Input: part model. Units: mm. Frame: model coordinates. Round coordinates to 2 decimals unless told otherwise and drop trailing zeros. Loops run counter-clockwise (first coordinate to the right, second up) from the corner with the lowest first, then second, coordinate; pieces in that order, holes last.
(1) Cut plane A-A, the plane y = 25. Output: boundary loops of the cut face in (x, z).
(2) First-contact query: pin 1 Ø4 at (y, z) = (25, 0) entering from -X; pin 2 Ø5 at (y, z) = (5, 0) entering from +X. Flat tips, straight axial feed; report the tip coordinate or a pass-through.
(3) Line query: line 1 (Y direction, x = 0, z = 4.25); line 2 (Y direction, x = -4.5, z = 0); line 3 (Z direction, x = 2.25, y = 66.5). Output: solid intervals per line, ascending.
(4) Cut plane C-C, the plane x = 0. Output: boundary loops of the cut face in (y, z), and give its area (3 significant figures).
(5) Cut plane B-B, the plane z = 0. Output: boundary loops of the cut face in (x, y), and give its area (3 significant figures).
(6) Cut plane D-D, the plane y = 114. Output: boundary loops of the cut face in (x, z).
from build123d import *

# Parameters (mm, degrees)
SKETCH_1_W          = 10
SKETCH_1_H          = 10
SKETCH_1_W_2        = 7
SKETCH_1_H_2        = 7
EXTRUDE_1_DEPTH     = 220
SKETCH_2_R          = 2.15
CUT_EXTRUDE_1_DEPTH = 221.283907719
SKETCH_3_R          = 2.15
CUT_EXTRUDE_2_DEPTH = 221.283907719


with BuildPart() as part:
    # ｽｹｯﾁ1 → 押し出し-薄板1 (new body)
    with BuildSketch(Plane(origin=(0, 0, 0), x_dir=(1, 0, 0), z_dir=(0, 1, 0))):
        Rectangle(SKETCH_1_W, SKETCH_1_H)
        Rectangle(SKETCH_1_W_2, SKETCH_1_H_2, mode=Mode.SUBTRACT)
    extrude(amount=EXTRUDE_1_DEPTH)

    # ｽｹｯﾁ2 → ｶｯﾄ - 押し出し1 (cut, through all)
    with BuildSketch(Plane.XY.offset(5)):
        with Locations((0, 205)):
            Circle(SKETCH_2_R)
        with Locations((0, 215)):
            Circle(SKETCH_2_R)
    extrude(amount=-CUT_EXTRUDE_1_DEPTH, mode=Mode.SUBTRACT)

    # ｽｹｯﾁ3 → ｶｯﾄ - 押し出し2 (cut, through all)
    with BuildSketch(Plane(origin=(5, 0, 0), x_dir=(0, 0, -1), z_dir=(1, 0, 0))):
        with Locations((0, 5)):
            Circle(SKETCH_3_R)
        with Locations((0, 25)):
            Circle(SKETCH_3_R)
    extrude(amount=-CUT_EXTRUDE_2_DEPTH, mode=Mode.SUBTRACT)


solid = part.part
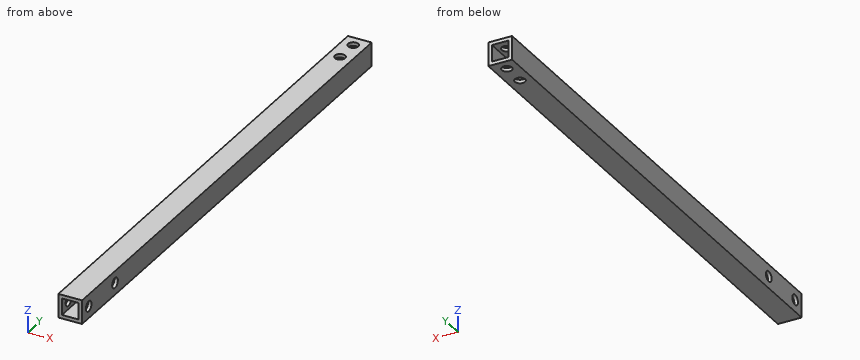
Reported:
1. outline: (-5, -5) - (5, -5) - (5, -2.15) - (3.5, -2.15) - (3.5, -3.5) - (-3.5, -3.5) - (-3.5, -2.15) - (-5, -2.15) - close; (-5, 2.15) - (-3.5, 2.15) - (-3.5, 3.5) - (3.5, 3.5) - (3.5, 2.15) - (5, 2.15) - (5, 5) - (-5, 5) - close
2. pin 1: passes through
2. pin 2: stops at x = 5
3. line 1: y = 0 to 202.85, 207.15 to 212.85, 217.15 to 220
3. line 2: y = 0 to 2.85, 7.15 to 22.85, 27.15 to 220
3. line 3: z = -5 to -3.5, 3.5 to 5
4. outline: (0, -5) - (202.85, -5) - (202.85, -3.5) - (0, -3.5) - close; (0, 3.5) - (202.85, 3.5) - (202.85, 5) - (0, 5) - close; (207.15, -5) - (212.85, -5) - (212.85, -3.5) - (207.15, -3.5) - close; (207.15, 3.5) - (212.85, 3.5) - (212.85, 5) - (207.15, 5) - close; (217.15, -5) - (220, -5) - (220, -3.5) - (217.15, -3.5) - close; (217.15, 3.5) - (220, 3.5) - (220, 5) - (217.15, 5) - close
4. area: 634 mm2
5. outline: (-5, 0) - (-3.5, 0) - (-3.5, 2.85) - (-5, 2.85) - close; (-5, 7.15) - (-3.5, 7.15) - (-3.5, 22.85) - (-5, 22.85) - close; (-5, 27.15) - (-3.5, 27.15) - (-3.5, 220) - (-5, 220) - close; (3.5, 0) - (5, 0) - (5, 2.85) - (3.5, 2.85) - close; (3.5, 7.15) - (5, 7.15) - (5, 22.85) - (3.5, 22.85) - close; (3.5, 27.15) - (5, 27.15) - (5, 220) - (3.5, 220) - close
5. area: 634 mm2
6. outline: (-5, -5) - (5, -5) - (5, 5) - (-5, 5) - close; hole (-3.5, -3.5) - (3.5, -3.5) - (3.5, 3.5) - (-3.5, 3.5) - close
